from build123d import *

# Parameters (mm, degrees)
F2_R            = 3.5
F3_DEPTH        = 4
F4_D            = 2.5
F4_CBORE_D      = 4.5
F4_CBORE_DEPTH  = 2
F5_DEPTH        = 15
F7_D            = 3
F7_DEPTH        = 13.5
F7_CSINK_D      = 4
F7_CSINK_ANGLE  = 90
F7_TIP          = 0.9012909285
F9_D            = 3
F9_DEPTH        = 13.5
F9_CSINK_D      = 4
F9_CSINK_ANGLE  = 90
F9_TIP          = 0.9012909285
F11_D           = 3
F11_DEPTH       = 13.5
F11_CSINK_D     = 4
F11_CSINK_ANGLE = 90
F11_TIP         = 0.9012909285
F13_D           = 3
F13_DEPTH       = 13.5
F13_CSINK_D     = 4
F13_CSINK_ANGLE = 90
F13_TIP         = 0.9012909285


with BuildPart() as f3:
    # F2 (on Top) → F3 (new body)
    with BuildSketch(Plane.XY):
        Polygon((27.5709562153, 77.495081059), (-22.4290437847, 77.495081059), (-22.4290437847, 73.495081059), (-22.4290437847, -18.5049188996), (-22.4290437847, -22.504918941), (27.5709562153, -22.504918941), (27.5709562153, -18.504918941), (27.5709562153, 73.495081059), align=None)
        with BuildLine():
            ThreePointArc((-15.4290437847, -18.504918941), (-18.9290438054, -22.004918941), (-22.4290437847, -18.5049188996))
            ThreePointArc((-22.4290437847, -18.5049188996), (-18.9290437641, -15.004918941), (-15.4290437847, -18.504918941))
        make_face(mode=Mode.SUBTRACT)
        with Locations((24.0709562153, -18.504918941)):
            Circle(F2_R, mode=Mode.SUBTRACT)
        with BuildLine():
            ThreePointArc((-15.4290437847, 73.495081059), (-18.9290437847, 69.995081059), (-22.4290437847, 73.495081059))
            ThreePointArc((-22.4290437847, 73.495081059), (-18.9290437847, 76.995081059), (-15.4290437847, 73.495081059))
        make_face(mode=Mode.SUBTRACT)
        with Locations((24.0709562153, 73.495081059)):
            Circle(F2_R, mode=Mode.SUBTRACT)
        with BuildLine():
            ThreePointArc((-15.4290437847, -18.504918941), (-18.9290437641, -15.004918941), (-22.4290437847, -18.5049188996))
            ThreePointArc((-22.4290437847, -18.5049188996), (-18.9290438054, -22.004918941), (-15.4290437847, -18.504918941))
        make_face()
        with Locations((24.0709562153, -18.504918941)):
            Circle(F2_R)
        with BuildLine():
            ThreePointArc((-15.4290437847, 73.495081059), (-18.9290437847, 76.995081059), (-22.4290437847, 73.495081059))
            ThreePointArc((-22.4290437847, 73.495081059), (-18.9290437847, 69.995081059), (-15.4290437847, 73.495081059))
        make_face()
        with Locations((24.0709562153, 73.495081059)):
            Circle(F2_R)
    extrude(amount=F3_DEPTH)

    # F4 (through all)
    with Locations(Plane(origin=(0, 0, 0), x_dir=(1, 0, 0), z_dir=(0, 0, -1))):
        with Locations((19.5709562153, -69.995081059), (19.5709562153, 15.004918941), (-14.4290437847, 15.004918941), (-14.4290437847, -69.995081059)):
            CounterBoreHole(F4_D / 2, F4_CBORE_D / 2, F4_CBORE_DEPTH)

    # F2 (on Top) → F5 (join)
    with BuildSketch(Plane.XY):
        with BuildLine():
            ThreePointArc((-15.4290437847, -18.504918941), (-18.9290437641, -15.004918941), (-22.4290437847, -18.5049188996))
            ThreePointArc((-22.4290437847, -18.5049188996), (-18.9290438054, -22.004918941), (-15.4290437847, -18.504918941))
        make_face()
        with Locations((24.0709562153, -18.504918941)):
            Circle(F2_R)
        with BuildLine():
            ThreePointArc((-15.4290437847, 73.495081059), (-18.9290437847, 76.995081059), (-22.4290437847, 73.495081059))
            ThreePointArc((-22.4290437847, 73.495081059), (-18.9290437847, 69.995081059), (-15.4290437847, 73.495081059))
        make_face()
        with Locations((24.0709562153, 73.495081059)):
            Circle(F2_R)
    extrude(amount=-F5_DEPTH)

    # F7
    with Locations(Plane(origin=(0, 0, -15), x_dir=(1, 0, 0), z_dir=(0, 0, -1))):
        with Locations((-18.9290437847, -73.495081059)):
            CounterSinkHole(F7_D / 2, F7_CSINK_D / 2, depth=F7_DEPTH, counter_sink_angle=F7_CSINK_ANGLE)
            with Locations((0, 0, -(F7_DEPTH + F7_TIP / 2))):  # 118° drill point
                Cone(0, F7_D / 2, F7_TIP, mode=Mode.SUBTRACT)

    # F9
    with Locations(Plane(origin=(0, 0, -15), x_dir=(1, 0, 0), z_dir=(0, 0, -1))):
        with Locations((-18.9290437847, 18.504918941)):
            CounterSinkHole(F9_D / 2, F9_CSINK_D / 2, depth=F9_DEPTH, counter_sink_angle=F9_CSINK_ANGLE)
            with Locations((0, 0, -(F9_DEPTH + F9_TIP / 2))):  # 118° drill point
                Cone(0, F9_D / 2, F9_TIP, mode=Mode.SUBTRACT)

    # F11
    with Locations(Plane(origin=(0, 0, -15), x_dir=(1, 0, 0), z_dir=(0, 0, -1))):
        with Locations((24.0709562153, -73.495081059)):
            CounterSinkHole(F11_D / 2, F11_CSINK_D / 2, depth=F11_DEPTH, counter_sink_angle=F11_CSINK_ANGLE)
            with Locations((0, 0, -(F11_DEPTH + F11_TIP / 2))):  # 118° drill point
                Cone(0, F11_D / 2, F11_TIP, mode=Mode.SUBTRACT)

    # F13
    with Locations(Plane(origin=(0, 0, -15), x_dir=(1, 0, 0), z_dir=(0, 0, -1))):
        with Locations((24.0709562153, 18.504918941)):
            CounterSinkHole(F13_D / 2, F13_CSINK_D / 2, depth=F13_DEPTH, counter_sink_angle=F13_CSINK_ANGLE)
            with Locations((0, 0, -(F13_DEPTH + F13_TIP / 2))):  # 118° drill point
                Cone(0, F13_D / 2, F13_TIP, mode=Mode.SUBTRACT)


solid = f3.part
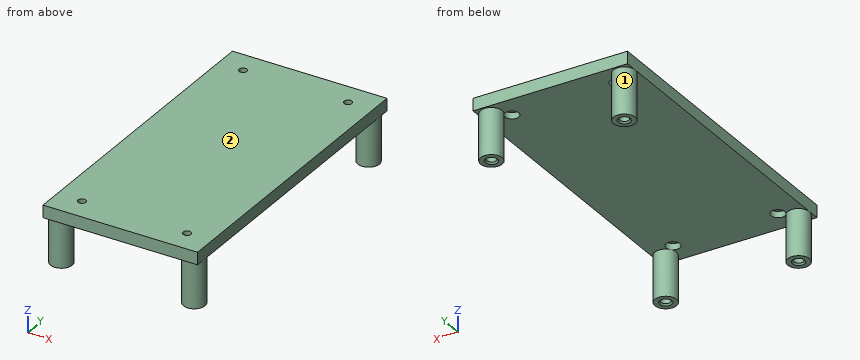
Part model, mm, in its own coordinate system. Face numbers are marked on the shaded views. Coordinates: 2 decimals unless noted, no trailing zeros. Order: outer loops, then holes, each group sorted by start corner. A loop starts at its lowest first (then second) coordinate and runs counter-clockwise, first axis right, second up.
(1) Slice it at C-C, the plane y = 26.5. Write the cut outline in (x, z), and give its area (3 significant figures).
Check sheet entries:
outline: (-22.43, 0) - (27.57, 0) - (27.57, 4) - (-22.43, 4) - close
area: 200 mm2
(2) Slice it at B-B, the plane x = 7. Write the cut outline in (y, z).
Check sheet entries:
outline: (-22.5, 0) - (77.5, 0) - (77.5, 4) - (-22.5, 4) - close
(3) Pin check, flat tips, straight feed: pin 1 Ø12 at (x, y) = (6.5, 8.5) entering from -Z; pin 2 Ø1.3 at (x, y) = (-15, -15.5) entering from -Z; pin 3 Ø5 at (x, y) = (-14.43, -15) entering from -Z; pin 4 Ø2.5 at (x, y) = (24.07, -18.5) entering from -Z. Stop position of each tip, or through.
Check sheet entries:
pin 1: stops at z = 0
pin 2: stops at z = 2
pin 3: stops at z = -15
pin 4: stops at z = -1.35
(4) Slice it at A-A, the plane z = -2.5. Write the cut outline in (x, y), and give its area (3 significant figures).
Check sheet entries:
outline: circle Ø7 at (-18.93, -18.5); circle Ø7 at (-18.93, 73.5); circle Ø7 at (24.07, -18.5); circle Ø7 at (24.07, 73.5); hole circle Ø3 at (-18.93, -18.5); hole circle Ø3 at (-18.93, 73.5); hole circle Ø3 at (24.07, -18.5); hole circle Ø3 at (24.07, 73.5)
area: 126 mm2
(5) Pull direction X, two halves, no side cores. Call the marked faces 1 and 2: pulls with the +X half, pulls with the -X half, needs draft (parallel to the pull), parting line crosses it, or undercut.
Check sheet entries:
face 1: undercut
face 2: needs draft
(6) Probe L1, parallel to Y at x = 24, z = -9.5; L2, parallel to Y at x = 23.5, z = -7; L3, parallel to Z at x = -12, y = 51. List the from-to ranges inside material, lowest first.
Check sheet entries:
L1: y = -22 to -20, -17.01 to -15.01, 70 to 72, 74.99 to 76.99
L2: y = -21.96 to -19.89, -17.12 to -15.05, 70.04 to 72.11, 74.88 to 76.95
L3: z = 0 to 4
